Part model, mm, in its own coordinate system. Face numbers are marked on the shaded views. A direction names the side the tool comes from. Round coordinates to 2 decimals unless told otherwise and drop trailing zeros. Write each loop counter-clockwise with the first axis right and the second up, starting at its lowest first coordinate (ties: lowest second). Pieces come first, ordered by that corner, then holes. Notation, with made-up numbers: M 40,86.25 L 61,86.25 A19 cw 61,99.25 Z; hole C 53.5,36 d8. An arc over 180 degrees is marked long. Use one line per item in the form item = value. Start each with the question number.
Item 1: Flat gauge pins, fed straight in: pin 1 Ø2 at (x, z) = (-15, 0.5) entering from -Y; pin 2 Ø3 at (y, z) = (34, 0) entering from +X; pin 3 Ø4 at (x, y) = (-16, 31) entering from +Z. Where does each tip first touch, or does it go through?
Item 2: Mould opens along Y. For the marked faces 1, 2, 3 and 4 say: +Y half, -Y half, draft (parallel to the pull), parting line (faces both ways), or undercut.
Item 3: Cut at B-B, the plane z = 0. Give the cut face in (x, y).
Item 4: Cut at C-C, the plane x = -23. Give the cut face in (y, z).
Item 5: Probe L1, parallel to Y at x = -21.9, z = 0; L2, parallel to Y at x = -17.5, z = -2.5; L3, parallel to Z at x = -23.1, y = 23.75. List the from-to ranges inside material, lowest first.
Item 6: Cut at A-A, the plane x = -15.25. Give the cut face in (y, z), then the cut area to 3 significant figures.
Item 7: Cut at D-D, the plane y = 23.75. Give the cut face in (x, z).
Item 8: Which spindle directions (+Z, -Z, +X, -X, +Y, -Y) get a long thin tool onto all of the face, cutting with end or side? Do the marked faces 5, 6, 7 and 8. Say none if no direction does.
from build123d import *

# Parameters (mm, degrees)
SKETCH009_R               = 1.25
EXTRUDE006_DEPTH          = 1.6
SKETCH007_R               = 1.25
EXTRUDE004_DEPTH          = 11
EXTRUDE003_DEPTH          = 3.3
FUSION021_ROLL_ANGLE      = -90
FUSION021_PLACEMENT_ANGLE = -90


with BuildPart() as opticalsensorpcbonlyonetab:
    # Sketch009 → Extrude006 (new body)
    with BuildSketch(Plane.XY):
        with BuildLine():
            Line((-6, 0), (6, 0))
            Line((6, 0), (6, 8))
            Line((6, 8), (9.75, 8))
            ThreePointArc((9.75, 8), (13, 11.25), (9.75, 14.5))
            Line((-7, 14.5), (9.75, 14.5))
            Line((-7, 8), (-7, 14.5))
            Line((-6, 8), (-7, 8))
            Line((-6, 0), (-6, 8))
        make_face()
        with Locations((10.25, 11.25)):
            Circle(SKETCH009_R, mode=Mode.SUBTRACT)
    extrude(amount=EXTRUDE006_DEPTH)


with BuildPart() as obj1:
    # Sketch007 → Extrude004 (new body)
    with BuildSketch(Plane.XY):
        with BuildLine():
            Line((-7, 3.25), (9.75, 3.25))
            ThreePointArc((9.75, -3.25), (13, 0), (9.75, 3.25))
            Line((-7, -3.25), (9.75, -3.25))
            Line((-7, -3.25), (-7, 3.25))
        make_face()
        with Locations((10.25, 0)):
            Circle(SKETCH007_R, mode=Mode.SUBTRACT)
    extrude(amount=EXTRUDE004_DEPTH)


with BuildPart() as obj2:
    # Sketch006 → Extrude003 (new body, symmetric)
    with BuildSketch(Plane.XZ):
        Polygon((-7, 0), (13, 0), (13, 2.7), (7, 2.7), (7, 11), (3, 11), (3, 2.7), (-3, 2.7), (-3, 11), (-7, 11), align=None)
    extrude(amount=EXTRUDE003_DEPTH, both=True)

    # Common: intersect obj1
    add(obj1.part, mode=Mode.INTERSECT)


with BuildPart() as obj2_1:
    # Common placement: moved
    add(obj2.part.moved(Location((0, 11.25, 1.6))))

    # Fusion021: union OpticalSensorPcbOnlyOneTab
    add(opticalsensorpcbonlyonetab.part)


with BuildPart() as obj2_2:
    # Fusion021 roll: moved
    add(obj2_1.part.rotate(Axis((0, 0, 0), (1, 0, 0)), FUSION021_ROLL_ANGLE))


with BuildPart() as obj2_3:
    # Fusion021 placement: moved
    add(obj2_2.part.moved(Location((-24, 34, 11.25))).rotate(Axis((-24, 34, 11.25), (0, 0, 1)), FUSION021_PLACEMENT_ANGLE))


solid = obj2_3.part
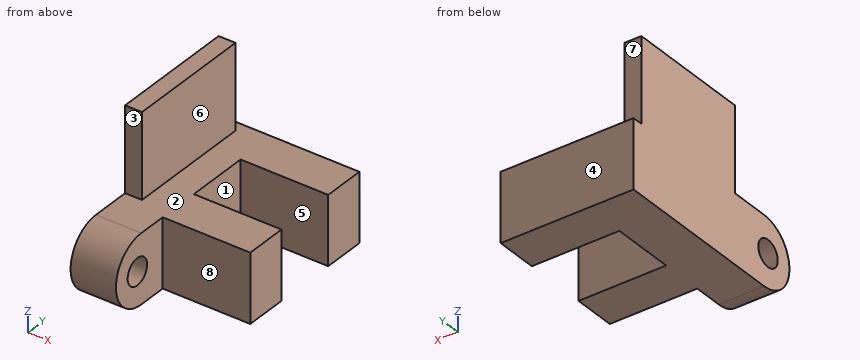
Model answer:
q1.pin_1 = 27
q1.pin_2 = -19.7
q1.pin_3 = 3.25
q2.face_1 = undercut
q2.face_2 = draft
q2.face_3 = -Y half
q2.face_4 = +Y half
q3.outline = M -24,21 L -19.7,21 L -19.7,22.5 L -24,22.5 Z; M -24,25 L -19.7,25 L -19.7,27 L -11.4,27 L -11.4,31 L -19.7,31 L -19.7,37 L -11.4,37 L -11.4,41 L -24,41 Z
q4.outline = M 24.25,-3.25 L 41,-3.25 L 41,3.25 L 40,3.25 L 40,11.25 L 28,11.25 L 28,3.25 L 24.25,3.25 A3.25 ccw Z; hole C 23.75,0 d2.5
q5.L1 = 21 to 22.5, 25 to 41
q5.L2 = 27 to 31, 37 to 41
q5.L3 = -3.21 to -1.25, 1.25 to 3.21
q6.outline = M 27,-3.25 L 31,-3.25 L 31,3.25 L 27,3.25 Z; M 37,-3.25 L 41,-3.25 L 41,3.25 L 37,3.25 Z
q6.area = 52.0 mm²
q7.outline = M -24,-3.21 L -19.7,-3.21 L -19.7,-1.25 L -24,-1.25 Z; M -24,1.25 L -19.7,1.25 L -19.7,3.21 L -24,3.21 Z
q8.face_5 = +Z, -Z, +X
q8.face_6 = +Z, +X, +Y, -Y
q8.face_7 = +Z, +X, -X, +Y
q8.face_8 = +Z, -Z, +X, -Y
